from build123d import *

# Parameters (mm, degrees)
FILLET_2_R          = 2.5
CUT_EXTRUDE_2_DEPTH = 4.5
SKETCH_6_R          = 7.544495516
SKETCH_6_R_2        = 6.742597779
EXTRUDE_2_DEPTH     = 7.9
SKETCH_7_R          = 15
EXTRUDE_3_DEPTH     = 10
CHAMFER_1_SIZE      = 0.5
SKETCH_8_R          = 13.5
EXTRUDE_4_DEPTH     = 7
SKETCH_9_R          = 14.25
EXTRUDE_5_DEPTH     = 6
CHAMFER_2_SIZE      = 1
SKETCH_10_R         = 11
EXTRUDE_6_DEPTH     = 7
SKETCH_11_W         = 46
SKETCH_11_H         = 30
EXTRUDE_7_DEPTH     = 36
FILLET_3_R          = 2.5


with BuildPart() as part:
    # Эскиз2 → Повернуть1 (revolve)
    with BuildSketch(Plane.XY, mode=Mode.PRIVATE) as revolve_1_sk:
        with BuildLine():
            Line((0, 2.930948498), (20, 2.930948498))
            Line((20, 2.930948498), (20, 7.930948498))
            add(Edge.make_bspline(
                [(20, 7.930948498), (10.236656465, 11.004873072), (0, 10.930948498)],
                knots=[0, 0, 0, 1, 1, 1], degree=2))
            Line((0, 10.930948498), (0, 2.930948498))
        make_face()
    revolve(revolve_1_sk.sketch.rotate(Axis((0, 45.754032666, 0), (0, -1, 0)), 90), axis=Axis((0, 45.754032666, 0), (0, -1, 0)))

    # Скругление2
    fillet_2_edges = [part.edges().sort_by_distance(p)[0] for p in [
        (0, 2.930948498, -20),
        (0, 7.930948498, -20),
    ]]
    fillet(fillet_2_edges, radius=FILLET_2_R)

    # Эскиз5 → Вырез-Вытянуть2 (cut)
    with BuildSketch(Plane(origin=(0, 13.812870775, 0), x_dir=(1, 0, 0), z_dir=(0, 1, 0))):
        with BuildLine():
            Line((-13.616818713, 2.867646528), (-12.134990634, 3.590023912))
            Line((-12.134990634, 3.590023912), (-11.048077198, 2.326680033))
            ThreePointArc((-11.048077198, 2.326680033), (-0.317231994, 11.285956477), (10.899937011, 2.943607126))
            Line((10.899937011, 2.943607126), (12.486323695, 2.058637888))
            Line((12.486323695, 2.058637888), (13.476651449, 3.467133424))
            ThreePointArc((13.476651449, 3.467133424), (-0.307827631, 13.91209512), (-13.616818713, 2.867646528))
        make_face()
        with BuildLine():
            Line((11.046374652, -2.334749837), (12.066615041, -3.813537836))
            Line((12.066615041, -3.813537836), (13.616818713, -2.867646528))
            ThreePointArc((13.616818713, -2.867646528), (0.349599989, -13.911108091), (-13.455587055, -3.548003025))
            Line((-13.455587055, -3.548003025), (-12.486323695, -2.058637888))
            Line((-12.486323695, -2.058637888), (-10.917619437, -2.877331328))
            ThreePointArc((-10.917619437, -2.877331328), (0.278824577, -11.286970657), (11.046374652, -2.334749837))
        make_face()
    extrude(amount=-CUT_EXTRUDE_2_DEPTH, mode=Mode.SUBTRACT)

    # Эскиз6 → Бобышка-Вытянуть2 (add)
    with BuildSketch(Plane.XZ.offset(-2.930948498)):
        with Locations(Location((0, 0, 0), (0, 0, 270))):
            Circle(SKETCH_6_R)
        with Locations(Location((0, 0, 0), (0, 0, 270))):
            Circle(SKETCH_6_R_2, mode=Mode.SUBTRACT)
    extrude(amount=-EXTRUDE_2_DEPTH)

    # Эскиз7 → Бобышка-Вытянуть3 (add)
    with BuildSketch(Plane.XZ.offset(-2.930948498)):
        with Locations(Location((0, 0, 0), (0, 0, 90))):
            Circle(SKETCH_7_R)
    extrude(amount=EXTRUDE_3_DEPTH)

    # Фаска1
    chamfer_1_edges = [part.edges().sort_by_distance(p)[0] for p in [
        (0, -7.069051502, -15),
    ]]
    chamfer(chamfer_1_edges, length=CHAMFER_1_SIZE)

    # Эскиз8 → Бобышка-Вытянуть4 (add)
    with BuildSketch(Plane.XZ.offset(7.069051502)):
        with Locations(Location((0, 0, 0), (0, 0, 270))):
            Circle(SKETCH_8_R)
    extrude(amount=EXTRUDE_4_DEPTH)

    # Эскиз9 → Бобышка-Вытянуть5 (add)
    with BuildSketch(Plane.XZ.offset(14.069051502)):
        with Locations(Location((0, 0, 0), (0, 0, 270))):
            Circle(SKETCH_9_R)
    extrude(amount=EXTRUDE_5_DEPTH)

    # Фаска2
    # the kernel refuses this chamfer: 1 mm, written as the material it adds along each edge
    with BuildSketch(Plane(origin=(0, -14.069051502, 0), x_dir=(0, 0, -1), z_dir=(-1, 0, 0))) as chamfer_2_piece_1_section:
        Polygon((13.5 + CHAMFER_2_SIZE, 0), (13.5, -CHAMFER_2_SIZE), (13.5, 0), align=None)
    chamfer_2_piece_1 = revolve(axis=Axis((0, -14.069051502, 0), (0, -1, 0)), mode=Mode.PRIVATE)
    chamfer_2_piece_1 = chamfer_2_piece_1 & Plane(origin=(0, -13.454886429, 0), x_dir=(0, 0, -1), z_dir=(0, 1, 0)) * Cylinder(14.25, 58, mode=Mode.PRIVATE)
    add(chamfer_2_piece_1)

    # Эскиз10 → Бобышка-Вытянуть6 (add)
    with BuildSketch(Plane.XZ.offset(20.069051502)):
        with Locations(Location((0, 0, 0), (0, 0, 270))):
            Circle(SKETCH_10_R)
    extrude(amount=EXTRUDE_6_DEPTH)

    # Эскиз11 → Бобышка-Вытянуть7 (add)
    with BuildSketch(Plane.XZ.offset(27.069051502)):
        Rectangle(SKETCH_11_W, SKETCH_11_H)
    extrude(amount=EXTRUDE_7_DEPTH)

    # Скругление3
    fillet_3_edges = [part.edges().sort_by_distance(p)[0] for p in [
        (-23, -27.069051502, 0),
        (-23, -45.069051502, 15),
        (0, -27.069051502, -15),
        (-23, -45.069051502, -15),
        (23, -27.069051502, 0),
        (23, -45.069051502, -15),
        (0, -27.069051502, 15),
        (23, -45.069051502, 15),
        (-23, -63.069051502, 0),
        (0, -63.069051502, -15),
        (23, -63.069051502, 0),
        (0, -63.069051502, 15),
    ]]
    fillet(fillet_3_edges, radius=FILLET_3_R)


solid = part.part
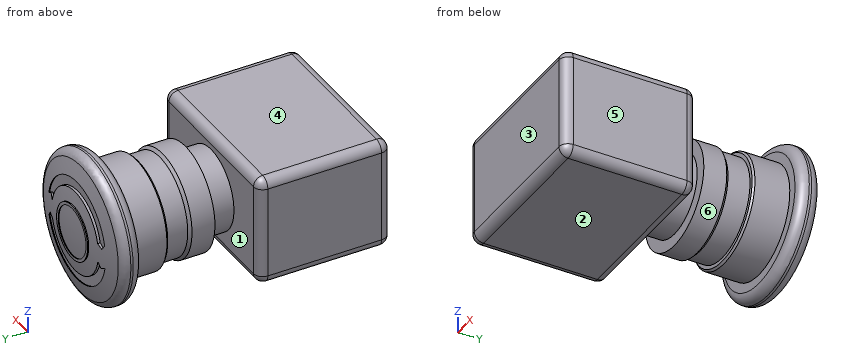
Model file for the job. Use its own axes, mm. Face numbers are marked on the shaded views. A direction names the side the tool comes from. Coordinates: 2 decimals unless noted, no trailing zeros. Write each loop counter-clockwise with the first axis right and the second up, starting at its lowest first coordinate (ties: lowest second). Pieces come first, ordered by that corner, then holes. Notation, with made-up numbers: (-16.5, 66.25) - (27.5, 66.25) arc R21 ccw to (27.5, 88.25) - close; hole circle Ø7 at (12, 79.25). An arc over 180 degrees is marked (long way). Write each question's results on one line, items separated by ' | '. Start each with the question number.
1) 3-axis set-ups, long thin cutter, end or side, ignore diameter. For the marked faces 4, 5 and 6: which of +Z, -Z, +X, -X, +Y, -Y reach the whole face in a straight line?
2) Flat gauge pins, fed straight in: P1, Ø5, axis at x = -8, y = -40, coming from the +Z side; P2, Ø5, axis at x = -9, y = -25.5, coming from the +Z side; P3, Ø2, axis at y = -3, z = -13, coming from the -X side; P4, Ø4, axis at x = 17, y = -22, coming from the -Z side. Where does each tip first touch, or does it go through?
3) Cut at A-A (y = -39.5). Write the cut outline in (x, z), then the cut area to 3 significant figures.
4) Mould opens along Y. For the marked faces 1, 2 and 3 say: pulls with the +Y half, pulls with the -Y half, needs draft (parallel to the pull), parting line crosses it, or undercut.
5) Cut at B-B (y = -8.5). Write the cut outline in (x, z).
6) Probe line 1 along Y through (x, z) = (-1, 11.5); line 2 along Y through (x, z) = (9, -12.5); line 3 along Z through (x, y) = (0, 10). List the from-to ranges inside material, lowest first. Write a range as from..to.
Returned:
1) face 4: +Z, +X, -X, -Y | face 5: +Z, -Z, +X, +Y, -Y | face 6: none
2) P1: z = 15 | P2: z = 14.45 | P3: x = -9 | P4: through
3) outline: (-23, -12.5) arc R2.5 ccw to (-20.5, -15) - (20.5, -15) arc R2.5 ccw to (23, -12.5) - (23, 12.5) arc R2.5 ccw to (20.5, 15) - (-20.5, 15) arc R2.5 ccw to (-23, 12.5) - close | area: 1,370 mm^2
4) face 1: undercut | face 2: needs draft | face 3: pulls with the -Y half
5) outline: circle Ø27 at (0, 0)
6) line 1: -63.07..-27.07, -20.07..9.31 | line 2: -63.07..-27.07, 2.93..9.2 | line 3: -11.29..11.29
